CAD build for the part. Positions are in the model's coordinates, mm. A direction names the side the tool comes from. Give positions to 0.01 mm unless a question says otherwise; leave off trailing zeros. Order: outer loops, then holes, each group sorted by start corner. A loop starts at its lowest first (then second) coordinate and runs counter-clockwise, first axis right, second up.
from build123d import *

# Parameters (mm, degrees)
F1_DEPTH = 25.4
F3_D     = 2.794
F3_DEPTH = 25.4
F3_TIP   = 0.8394022848
F4_D     = 2.794
F4_DEPTH = 25.4
F4_START = 10.1278152
F4_TIP   = 0.8394022848
F5_R     = 18.0883597705
F6_R     = 5.08


# Not quite as in the source:
# - ends of sketch curves that miss each other by under 0.0002 mm in the source are joined
# - a feature names something its author has since deleted; it is built from what else it names


with BuildPart() as f1:
    # F0 (on Front) → F1 (new body)
    with BuildSketch(Plane.XZ):
        Polygon((11.0066256276, -6.5430273301), (8.240193387, -9.310965985), (12.5485987193, -9.310965985), (12.5485987193, -1.1086727812), (9.7906497979, 6.8444932552), (24.9488617122, 22.0027051695), (31.3820510637, 28.435894521), (29.2404852808, 30.5774603039), (22.8072959293, 24.1442709524), (16.0729033236, 30.8786635582), (22.3196721338, 37.1254323684), (20.2273843878, 39.2177201144), (14.0302290969, 33.0205648235), (13.9806155776, 32.9709513042), (-7.4406042695, 11.5497314571), (-11.6305711889, -1.2286720797), (-11.6305711889, -9.3063699081), (-7.3613829189, -9.3063699081), (-10.1278151595, -6.5384312532), (-7.4425795762, -3.8636476732), (8.3167760077, -3.8636476732), align=None)
    extrude(amount=F1_DEPTH)

    # F3 (one way)
    with BuildSketch(Plane(origin=(0, 0, 0), x_dir=(0, 1, 0), z_dir=(-1, 0, 0))):
        with Locations((-22.1899207681, 6.5197679214), (-3.1917574815, 6.5197679214)):
            Circle(F3_D / 2)
    extrude(amount=-F3_DEPTH, mode=Mode.SUBTRACT)
    with Locations(Plane(origin=(0, 0, 0), x_dir=(0, 1, 0), z_dir=(-1, 0, 0))):
        with Locations((-22.1899207681, 6.5197679214), (-3.1917574815, 6.5197679214)):
            with Locations((0, 0, -(F3_DEPTH + F3_TIP / 2))):  # 118° drill point
                Cone(0, F3_D / 2, F3_TIP, mode=Mode.SUBTRACT)

    # F4
    # its depths count from where the whole tool has entered the part; down to there all is cleared
    with Locations(Plane.YZ.offset(-F4_START)):
        with Locations((-3.1917574815, -6.5197679214), (-22.1899207681, -6.5197679214)):
            Hole(F4_D / 2, depth=F4_DEPTH)
            with Locations((0, 0, -(F4_DEPTH + F4_TIP / 2))):  # 118° drill point
                Cone(0, F4_D / 2, F4_TIP, mode=Mode.SUBTRACT)

    # F5
    f5_edges = [f1.edges().sort_by_distance(p)[0] for p in [
        (-7.440604, -12.7, 11.549731),
    ]]
    fillet(f5_edges, radius=F5_R)

    # F6
    f6_edges = [f1.edges().sort_by_distance(p)[0] for p in [
        (9.79065, -12.7, 6.844493),
        (12.548599, -12.7, -1.108673),
    ]]
    fillet(f6_edges, radius=F6_R)


solid = f1.part
1. Wall check: line 1 (X direction, y = -18.25, z = -2); line 2 (Z direction, x = 10, y = -0.75); line 3 (X direction, y = -17.5, z = 30). Give the ranges that are in metal, low to high.
2. Pin check, flat tips, straight feed: P1, Ø2, axis at y = -19, z = 24, coming from the -X side; P2, Ø1.5, axis at y = -12, z = 31, coming from the +X side; P3, Ø2, axis at x = 3.5, y = -8.5, coming from the -Z side; P4, Ø12, axis at x = 24, y = -3, coming from the +Z side. Stop position of each tip, or through.
3. Saw through at C-C on x = -8. Give the cut face in (y, z), plus the area to 3 significant figures.
4. Mould opens along Y. For faces 1 (the flat face through (21.288, -12.522, 38.157)), 2 (the flat face through (8, -25.4, 13)), 3 (the cylindrical face through (11.365, -1.901, -5.985)), 4 (the cylindrical face through (-10.505, -22.008, -5.135)) say: released by +Y, released by -Y, zero draft, split by the parting line, or undercut.
5. Saw through at D-D on y = -22. Give the cut face in (x, z), plus the area to 3 significant figures.
6. Saw through at B-B on z = -4.5. Give the cut face in (x, y), plus the area to 3 significant figures.
7. Saw through at A-A on y = -17.5. Give the cut face in (x, z), plus the area to 3 significant figures.
8. 3-axis set-ups, long thin cutter, end or side, ignore diameter. For faces 5 (the flat face through (12.549, -13, -6)), 6 (the flat face through (-8.804, -12.522, -5.22)), 7 (the cylindrical face through (-7, -12.9, 11.3)), 8 (the flat face through (19.153, -12.522, 33.958)), 9 (the flat face through (0, -13, -3.864)): which of +Z, -Z, +X, -X, +Y, -Y reach the whole face in a straight line?
Reported:
1. line 1: x = -11.63 to 12.55
1. line 2: z = -9.31 to -7.55, -5.54 to 28.99
1. line 3: x = 11.01 to 16.95, 28.66 to 29.82
2. P1: stops at x = 4.01
2. P2: stops at x = 29.57
2. P3: stops at z = -3.86
2. P4: stops at z = 39.22
3. outline: (-25.4, -9.31) - (0, -9.31) - (0, -8.67) - (-25.4, -8.67) - close; (-25.4, -4.42) - (0, -4.42) - (0, 9.44) - (-25.4, 9.44) - close
3. area: 368 mm2
4. face 1: zero draft
4. face 2: released by -Y
4. face 3: undercut
4. face 4: undercut
5. outline: (-11.63, -9.31) - (-7.36, -9.31) - (-8.76, -7.9) - (-11.63, -7.9) - close; (-11.63, -5.14) - (-8.72, -5.14) - (-7.44, -3.86) - (8.32, -3.86) - (9.59, -5.14) - (12.55, -5.14) - (12.55, -1.96) arc R5.08 ccw to (12.27, -0.3) - (10.83, 3.84) arc R5.08 cw to (12.04, 9.09) - (31.38, 28.44) - (29.24, 30.58) - (22.81, 24.14) - (16.07, 30.88) - (22.32, 37.13) - (20.23, 39.22) - (-4.39, 14.6) arc R18.09 ccw to (-8.79, 7.45) - (-11.63, -1.23) - close; (8.24, -9.31) - (12.55, -9.31) - (12.55, -7.9) - (9.65, -7.9) - close
5. area: 756 mm2
6. outline: (-11.63, -25.4) - (-8.08, -25.4) - (-8.08, 0) - (-11.63, 0) - close; (8.96, -25.4) - (12.55, -25.4) - (12.55, 0) - (8.96, 0) - close
6. area: 181 mm2
7. outline: (-11.63, -9.31) - (-7.36, -9.31) - (-10.13, -6.54) - (-7.44, -3.86) - (8.32, -3.86) - (11.01, -6.54) - (8.24, -9.31) - (12.55, -9.31) - (12.55, -1.96) arc R5.08 ccw to (12.27, -0.3) - (10.83, 3.84) arc R5.08 cw to (12.04, 9.09) - (31.38, 28.44) - (29.24, 30.58) - (22.81, 24.14) - (16.07, 30.88) - (22.32, 37.13) - (20.23, 39.22) - (-4.39, 14.6) arc R18.09 ccw to (-8.79, 7.45) - (-11.63, -1.23) - close
7. area: 768 mm2
8. face 5: -Z, +X, +Y, -Y
8. face 6: +Y, -Y
8. face 7: +Z, -X, +Y, -Y
8. face 8: +X, +Y, -Y
8. face 9: -Z, +Y, -Y
